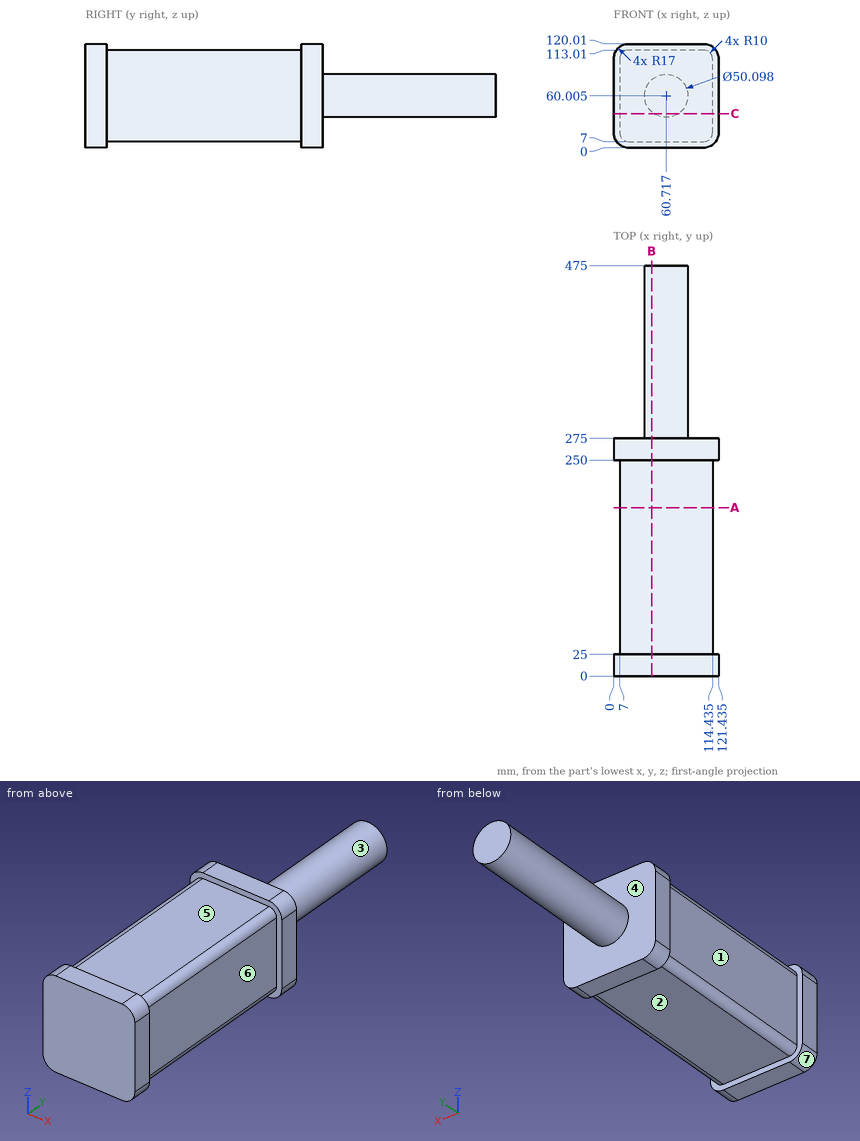
Geometry: see drawing. Coordinates: mm, zero at the bounding-box minimum. A direction names the side the tool comes from. Coordinates: 2 decimals unless noted, no trailing zeros. Order: outer loops, then holes, each group sorted by start corner. A loop starts at its lowest first (then second) coordinate and runs counter-clockwise, first axis right, second up. Notation, with made-up numbers: M 32,28 L 37,28 A6 ccw 37,39 Z; hole C 62.25,53 d9. An arc over 180 degrees is marked long. Answer in a Markdown table with one row per item. Add a question column.
Q1. Contact query for flat-ended pins moving along their axis: P1, Ø4, axis at y = 49.5, z = 76, coming from the +X side (1 decimal); P2, Ø12, axis at x = 49.5, y = 344, coming from the +Z side (1 decimal); P3, Ø12, axis at y = 382, z = 56, coming from the +X side. Output: stop coordinate, or through.
Q2. Section query A-A on y = 195. Return the cut outline in (x, z) (1 decimal), and give its area (3 significant figures).
Q3. Line query: L1, parallel to Y at x = 35, z = 55.5; L2, parallel to Z at x = 101.5, y = 62; L3, parallel to X at y = 185.5, z = 23 (1 decimal). Output: solid intervals per line, ascending.
Q4. Section query B-B on x = 44. Return the cut outline in (y, z).
Q5. Section query C-C on z = 39.5. Return the cut outline in (x, y) (1 decimal).
Q6. Reachability of the marked faces 1, 2 and 3 from +Z, -Z, +X, -X, +Y, -Y: full face, straight path, thin tool, end or side. Return the list, or none.
Q7. Mould query, pull axis Y, two halves, no side actions, for the marked faces 4, 5, 6 and 7. Classes: released by +Y, released by -Y, zero draft, split by the parting line, or undercut.
Completed:
| question | item | result |
|---|---|---|
| 1 | P1 | stops at x = 114.4 |
| 1 | P2 | stops at z = 84.5 |
| 1 | P3 | stops at x = 85.77 |
| 2 | outline | M 7,17 A10 ccw 17,7 L 104.4,7 A10 ccw 114.4,17 L 114.4,103 A10 ccw 104.4,113 L 17,113 A10 ccw 7,103 Z |
| 2 | area | 11,300 mm2 |
| 3 | L1 | y = 0 to 275 |
| 3 | L2 | z = 7 to 113.01 |
| 3 | L3 | x = 7 to 114.4 |
| 4 | outline | M 0,0 L 25,0 L 25,7 L 250,7 L 250,0 L 275,0 L 275,41.35 L 475,41.35 L 475,78.66 L 275,78.66 L 275,120.01 L 250,120.01 L 250,113.01 L 25,113.01 L 25,120.01 L 0,120.01 Z |
| 5 | outline | M 0,0 L 121.4,0 L 121.4,25 L 114.4,25 L 114.4,250 L 121.4,250 L 121.4,275 L 75.1,275 L 75.1,475 L 46.3,475 L 46.3,275 L 0,275 L 0,250 L 7,250 L 7,25 L 0,25 Z |
| 6 | face 1 | +Z, -Z, -X |
| 6 | face 2 | -Z, +X, -X |
| 6 | face 3 | +Y |
| 7 | face 4 | released by +Y |
| 7 | face 5 | undercut |
| 7 | face 6 | undercut |
| 7 | face 7 | zero draft |
